Read the model definition and answer for the solid it produces. Units are mm, in the model's axes. Face numbers are marked on the shaded views. A direction names the side the tool comes from. Give positions to 0.01 mm unless a question says otherwise; leave off trailing zeros. Order: outer loops, then holes, each group sorted by start corner. A loop starts at its lowest first (then second) coordinate and runs counter-clockwise, first axis right, second up.
```python
from build123d import *

# Parameters (mm, degrees)
SKETCH_1_R               = 40
EXTRUDE_1_DEPTH          = 100
SKETCH_2_R               = 35
CUT_EXTRUDE_1_DEPTH      = 92
SKETCH_3_R               = 35
EXTRUDE_2_DEPTH          = 8
SKETCH_4_W               = 3
SKETCH_4_H               = 11
EXTRUDE_3_DEPTH          = 92
PATTERN_CIRCULAR_1_COUNT = 12
SKETCH_5_R               = 11
CUT_EXTRUDE_2_DEPTH      = 8
SKETCH_6_R               = 3.5
CUT_EXTRUDE_3_DEPTH      = 8
SKETCH_7_R               = 2.25
CUT_EXTRUDE_4_DEPTH      = 8


with BuildPart() as part:
    # Sketch 1 → Extrude 1 (new body)
    with BuildSketch(Plane.XY):
        Circle(SKETCH_1_R)
    extrude(amount=EXTRUDE_1_DEPTH)

    # Sketch 2 → Cut-Extrude 1 (cut)
    with BuildSketch(Plane.XY.offset(8)):
        Circle(SKETCH_2_R)
    extrude(amount=CUT_EXTRUDE_1_DEPTH, mode=Mode.SUBTRACT)

    # Sketch 3 → Extrude 2 (add)
    with BuildSketch(Plane.XY.offset(92)):
        with BuildLine():
            Line((-40, -50), (40, -50))
            ThreePointArc((40, -50), (47.071067812, -47.071067812), (50, -40))
            Line((50, -40), (50, 40))
            ThreePointArc((50, 40), (47.071067812, 47.071067812), (40, 50))
            Line((40, 50), (-40, 50))
            ThreePointArc((-40, 50), (-47.071067812, 47.071067812), (-50, 40))
            Line((-50, 40), (-50, -40))
            ThreePointArc((-50, -40), (-47.071067812, -47.071067812), (-40, -50))
        make_face()
        Circle(SKETCH_3_R, mode=Mode.SUBTRACT)
    extrude(amount=EXTRUDE_2_DEPTH)

    # Sketch 4 → Extrude 3 (add)
    with BuildSketch(Plane.XY):
        with Locations((0, 44.5)):
            Rectangle(SKETCH_4_W, SKETCH_4_H)
    extrude_3 = extrude(amount=EXTRUDE_3_DEPTH)

    # Pattern Circular 1: Extrude 3 ×12 about axis
    pattern_circular_1_axis = Axis((0, 0, 0), (0, 0, 1))
    for i in range(1, PATTERN_CIRCULAR_1_COUNT):
        add(extrude_3.rotate(pattern_circular_1_axis, i * 360 / PATTERN_CIRCULAR_1_COUNT))

    # Sketch 5 → Cut-Extrude 2 (cut)
    with BuildSketch(Plane.XY):
        Circle(SKETCH_5_R)
    extrude(amount=CUT_EXTRUDE_2_DEPTH, mode=Mode.SUBTRACT)

    # Sketch 6 → Cut-Extrude 3 (cut)
    with BuildSketch(Plane.XY.offset(100)):
        with Locations((42, 42)):
            Circle(SKETCH_6_R)
        with Locations((-42, 42)):
            Circle(SKETCH_6_R)
        with Locations((-42, -42)):
            Circle(SKETCH_6_R)
        with Locations((42, -42)):
            Circle(SKETCH_6_R)
    extrude(amount=-CUT_EXTRUDE_3_DEPTH, mode=Mode.SUBTRACT)

    # Sketch 7 → Cut-Extrude 4 (cut)
    with BuildSketch(Plane.XY):
        with Locations((14.142136, 14.142136)):
            Circle(SKETCH_7_R)
        with Locations((-14.142136, 14.142136)):
            Circle(SKETCH_7_R)
        with Locations((-14.142136, -14.142136)):
            Circle(SKETCH_7_R)
        with Locations((14.142136, -14.142136)):
            Circle(SKETCH_7_R)
    extrude(amount=CUT_EXTRUDE_4_DEPTH, mode=Mode.SUBTRACT)


solid = part.part
```
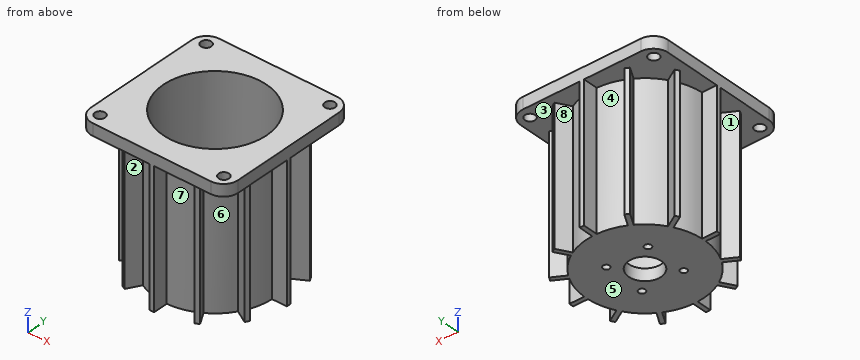
1) The part is cut by section A-A on y = 0. Determine the outline of the cut face in (x, z), and give its area (3 significant figures).
Final values:
outline: (-50, 0) - (-11, 0) - (-11, 8) - (-35, 8) - (-35, 100) - (-50, 100) - close; (11, 0) - (50, 0) - (50, 100) - (35, 100) - (35, 8) - (11, 8) - close
area: 3,380 mm2
2) The part is cut by section C-C on y = -29.5. Determine the outline of the cut face in (x, z).
Final values:
outline: (-50, 92) - (-27.01, 92) - (-27.01, 0) - (27.01, 0) - (27.01, 92) - (50, 92) - (50, 100) - (18.83, 100) - (18.83, 8) - (-18.83, 8) - (-18.83, 100) - (-50, 100) - close
3) A tool of negligible diameter and unlimited length cuts with its end or side. For the marked faces 1, 2, 3 and 4, from which of +Z, -Z, +X, -X, +Y, -Y can it reach the whole face along a straight path? Write none if from no direction.
Final values:
face 1: -Z, -X
face 2: -Z, -Y
face 3: -Z
face 4: -Z, +Y
4) Consider L1, parallel to Y at x = -42, z = 94; L2, parallel to Z at x = -40, y = 37; L3, parallel to X at y = 3.5, z = 77. Determine where each line is inside the solid, lowest interval first.
Final values:
L1: y = -49.8 to -45.5, -38.5 to 38.5, 45.5 to 49.8
L2: z = 92 to 100
L3: x = -39.85 to -34.82, 34.82 to 39.85
5) Given pin 1 (4 mm diameter, centred on x = -24, z = 47.5, fed in from -Y); pin 2 (5 mm diameter, centred on x = -46, z = 50.5, fed in from +Y); pin 3 (5 mm diameter, centred on x = 46, z = 45, fed in from -Y); pin 4 (6.5 mm diameter, centred on x = 42, y = 42, fed in from -Z), each flat-ended and moving along its own axis, determine where each tip first touches the part or whether it passes through.
Final values:
pin 1: stops at y = -44.05
pin 2: stops at y = 24.66
pin 3: stops at y = -24.66
pin 4: passes through
6) For a pull along Y with two mould halves and no side action, classify the marked faces 5, 6, 7 and 8 as released by +Y, released by -Y, zero draft, split by the parting line, or undercut.
Final values:
face 5: zero draft
face 6: undercut
face 7: released by -Y
face 8: released by +Y
